Geometry: final body of the model. Coordinates: model frame, mm. A direction names the side the tool comes from. Coordinates: 2 decimals unless noted, no trailing zeros. Write each loop counter-clockwise with the first axis right and the second up, starting at its lowest first coordinate (ties: lowest second). Pieces come first, ordered by that corner, then holes.
from build123d import *

# Parameters (mm, degrees)
F1_DEPTH = 15
F3_D     = 4.3
F3_DEPTH = 15
F3_TIP   = 1.2918503309
F4_R     = 5
F5_R     = 5
F7_DEPTH = 15.001
F9_D     = 4.3
F9_DEPTH = 20
F9_TIP   = 1.2918503309


with BuildPart() as f1:
    # F0 (on Front) → F1 (new body)
    with BuildSketch(Plane.XZ):
        Polygon((0, 100), (0, 0), (150, 0), (270, 0), (270, 30), (150, 100), align=None)
    extrude(amount=F1_DEPTH)

    # F3
    with Locations(Plane.XY.offset(100)):
        with Locations((125, -7.5), (75, -7.5), (25, -7.5)):
            Hole(F3_D / 2, depth=F3_DEPTH)
            with Locations((0, 0, -(F3_DEPTH + F3_TIP / 2))):  # 118° drill point
                Cone(0, F3_D / 2, F3_TIP, mode=Mode.SUBTRACT)

    # F4
    f4_edges = [f1.edges().sort_by_distance(p)[0] for p in [
        (270, -7.5, 30),
    ]]
    fillet(f4_edges, radius=F4_R)

    # F5
    f5_edges = [f1.edges().sort_by_distance(p)[0] for p in [
        (150, -7.5, 100),
    ]]
    fillet(f5_edges, radius=F5_R)

    # F6 (on Front) → F7 (cut, through all)
    with BuildSketch(Plane.XZ):
        Polygon((11.8321627378, 83.2323953509), (11.8321627378, 11.6192111745), (215.076940872, 11.6192111745), (215.076940872, 40.9227917323), (142.5461918116, 83.2323953509), align=None)
    extrude(amount=F7_DEPTH, mode=Mode.SUBTRACT)

    # F9
    with Locations(Plane(origin=(0, 0, 0), x_dir=(1, 0, 0), z_dir=(0, 0, -1))):
        with Locations((50, 7.5), (110, 7.5), (170, 7.5)):
            Hole(F9_D / 2, depth=F9_DEPTH)
            with Locations((0, 0, -(F9_DEPTH + F9_TIP / 2))):  # 118° drill point
                Cone(0, F9_D / 2, F9_TIP, mode=Mode.SUBTRACT)


solid = f1.part
Item 1: Pin query (flat end, axial travel): pin 1 (3 mm diameter, centred on y = -5, z = 58.5, fed in from +X); pin 2 (10 mm diameter, centred on x = 142.5, z = 20, fed in from -Y); pin 3 (3.5 mm diameter, centred on x = 125, y = -7.5, fed in from +Z). Return the tip coordinate at first contact, or that it passes through.
Derived:
pin 1: stops at x = 223.71
pin 2: passes through
pin 3: stops at z = 84.76
Item 2: Section B-B, the plane x = 34.5. Output: boundary loops of the cut face in (y, z), plus the area to 3 significant figures.
Derived:
outline: (-15, 0) - (0, 0) - (0, 11.62) - (-15, 11.62) - close; (-15, 83.23) - (0, 83.23) - (0, 100) - (-15, 100) - close
area: 426 mm2
Item 3: Pull-direction query (Z, two-part tool) for faces 3 (the flat face through (270, -7, 13)), 4 (the flat face through (112, -6, 11.619)), 5 (the flat face through (210, -7, 65)); classes: released by +Z, released by -Z, zero draft, split by the parting line, or undercut.
Derived:
face 3: zero draft
face 4: undercut
face 5: released by +Z
Item 4: Section C-C, the plane y = -2.5. Output: boundary loops of the cut face in (x, z).
Derived:
outline: (0, 0) - (270, 0) - (270, 27.13) arc R5 ccw to (267.52, 31.45) - (151.17, 99.32) arc R5 ccw to (148.65, 100) - (0, 100) - close; hole (11.83, 11.62) - (215.08, 11.62) - (215.08, 40.92) - (142.55, 83.23) - (11.83, 83.23) - close
Item 5: Set-up query: faces 1 (the flat face through (0, -7, 51)), 2 (the flat face through (215.077, -7, 26)). Return all of +Z, -Z, +X, -X, +Y, -Y with unobstructed straight access to the full face (end or side cutting, diameter ignored); none if empty.
Derived:
face 1: +Z, -Z, -X, +Y, -Y
face 2: +Y, -Y
Item 6: Section A-A, the plane z = 20. Output: boundary loops of the cut face in (x, y), plus the area to 3 significant figures.
Derived:
outline: (0, -15) - (11.83, -15) - (11.83, 0) - (0, 0) - close; (215.08, -15) - (270, -15) - (270, 0) - (215.08, 0) - close
area: 1,000 mm2
Item 7: Material intervals for probe 1 along X at (y, z) = (-7.5, 95); probe 2 along Z at (x, y) = (51.5, -13.75); probe 3 along X at (y, z) = (-7.5, 93), sorted ascending.
Derived:
probe 1: x = 0 to 22.85, 27.15 to 72.85, 77.15 to 122.85, 127.15 to 158.57
probe 2: z = 0 to 11.62, 83.23 to 100
probe 3: x = 0 to 22.85, 27.15 to 72.85, 77.15 to 122.85, 127.15 to 162
